For this review, take the finished solid that the model builds, in its own axes (mm). A direction names the side the tool comes from. Coordinates: 2 decimals unless noted, no trailing zeros. Order: outer loops, then holes, each group sorted by start corner. A loop starts at its lowest first (then second) coordinate and runs counter-clockwise, first axis right, second up.
from build123d import *

# Parameters (mm, degrees)
F1_DEPTH = 76.2
F2_R     = 12.7
F3_DEPTH = 76.201
F5_DEPTH = 25.401
F6_R     = 38.1
F9_DEPTH = 6.35


# Not quite as in the source:
# - a pattern or mirror of a feature is missing from the dataset's text; its kind, count and spacing are read off the source's solid


with BuildPart() as f1:
    # F0 (on Front) → F1 (new body, symmetric)
    with BuildSketch(Plane.XZ):
        Polygon((-76.2, 0), (0, 0), (0, 152.4), (-25.4, 152.4), (-25.4, 25.4), (-76.2, 25.4), align=None)
    extrude(amount=F1_DEPTH, both=True)

    # F2 (on Right) → F3 (cut, through all)
    with BuildSketch(Plane.YZ):
        with Locations((0, 114.3)):
            Circle(F2_R)
    extrude(amount=-F3_DEPTH, mode=Mode.SUBTRACT)

    # F4 (on face) → F5 (cut, through all)
    with BuildSketch(Plane.XY.offset(25.4)):
        with BuildLine():
            Line((-76.2, 12.7), (-76.2, 0))
            Line((-76.2, 0), (-76.2, -12.7))
            Line((-76.2, -12.7), (-63.5, -12.7))
            ThreePointArc((-63.5, -12.7), (-50.8, 0), (-63.5, 12.7))
            Line((-63.5, 12.7), (-76.2, 12.7))
        make_face()
    extrude(amount=-F5_DEPTH, mode=Mode.SUBTRACT)

    # F6
    f6_edges = [f1.edges().sort_by_distance(p)[0] for p in [
        (-12.7, -76.2, 152.4),
        (-12.7, 76.2, 152.4),
    ]]
    fillet(f6_edges, radius=F6_R)

    # F8 (on offset) → F9 (join, symmetric)
    with BuildSketch(Plane.XZ.offset(44.45)):
        Polygon((-50.8, 25.4), (-25.4, 25.4), (-25.4, 101.6), align=None)
    f9 = extrude(amount=F9_DEPTH, both=True)

    # F9_copies: F9 across plane
    add(f9.mirror(Plane.ZX))


solid = f1.part
1. Take a section at D-D, the plane z = 111.5. Give the boundary of the cut face in (x, y), plus the area to 3 significant figures.
Answer below:
outline: (-25.4, -76.2) - (0, -76.2) - (0, -12.39) - (-25.4, -12.39) - close; (-25.4, 12.39) - (0, 12.39) - (0, 76.2) - (-25.4, 76.2) - close
area: 3,240 mm2
2. Machinability: for faces 1 (the face through (-33, -50.8, 47)), 2 (the face through (-70, 12.7, 13)), 3 (the face through (-33, 38.1, 47)), which of the approach directions +Z, -Z, +X, -X, +Y, -Y give a long, thin tool a straight path to every point of the face, cutting with its end or side? Answer none if there is none.
Answer below:
face 1: +Z, -X, -Y
face 2: +Z, -Z, -X
face 3: +Z, -X
3. To check wall thickness, follow L1, parallel to Z at x = -9, y = 0; L2, parallel to Y at x = -38.5, z = 59; L3, parallel to X at y = 32.5, z = 62. State the ranges of each line that lie inside material, in increasing order.
Answer below:
L1: z = 0 to 101.6, 127 to 152.4
L2: y = -50.8 to -38.1, 38.1 to 50.8
L3: x = -25.4 to 0
4. Take a section at B-B, the plane x = -9. Give the boundary of the cut face in (y, z), plus the area to 3 significant figures.
Answer below:
outline: (-76.2, 0) - (76.2, 0) - (76.2, 114.3) arc R38.1 ccw to (38.1, 152.4) - (-38.1, 152.4) arc R38.1 ccw to (-76.2, 114.3) - close; hole circle Ø25.4 at (0, 114.3)
area: 22,100 mm2
5. The part is to be moulded in two halves that separate along Y. For faces 4 (the face through (-22, 76.2, 45)), 5 (the face through (-50, -1, 25.4)), 6 (the face through (-76.2, -45, 13)), say which applies: +Y half, -Y half, draft (parallel to the pull), parting line (faces both ways), or undercut.
Answer below:
face 4: +Y half
face 5: undercut
face 6: draft
6. Take a section at C-C, the plane z = 87.5. Give the boundary of the cut face in (x, y).
Answer below:
outline: (-30.1, -50.8) - (-25.4, -50.8) - (-25.4, -76.2) - (0, -76.2) - (0, 76.2) - (-25.4, 76.2) - (-25.4, 50.8) - (-30.1, 50.8) - (-30.1, 38.1) - (-25.4, 38.1) - (-25.4, -38.1) - (-30.1, -38.1) - close
7. Take a section at A-A, the plane y = 0. Give the boundary of the cut face in (x, z).
Answer below:
outline: (-50.8, 0) - (0, 0) - (0, 101.6) - (-25.4, 101.6) - (-25.4, 25.4) - (-50.8, 25.4) - close; (-25.4, 127) - (0, 127) - (0, 152.4) - (-25.4, 152.4) - close
8. Clearance check with flat-ended pins moving along their axes: pin 1 Ø8 at (x, y) = (-68.5, 57) entering from +Z; pin 2 Ø10 at (y, z) = (26, 30) entering from -X; pin 3 Ø4 at (x, z) = (-28, 41.5) entering from -Y; pin 4 Ø12.5 at (x, z) = (-41, 56) entering from +Y. State where each tip first meets the part, or that it passes through.
Answer below:
pin 1: stops at z = 25.4
pin 2: stops at x = -76.2
pin 3: stops at y = -50.8
pin 4: stops at y = 50.8
